from build123d import *

# Parameters (mm, degrees)
SKETCH1_W           = 47
SKETCH1_H           = 22
SKETCH1_R           = 5.25
BOSS_EXTRUDE1_DEPTH = 20
SKETCH2_R           = 10.5
SKETCH2_W           = 5.562030484
SKETCH2_H           = 6.723730134
CUT_EXTRUDE1_DEPTH  = 5


with BuildPart() as part:
    # Sketch1 → Boss-Extrude1 (new body)
    with BuildSketch(Plane.XY):
        Rectangle(SKETCH1_W, SKETCH1_H)
        Circle(SKETCH1_R, mode=Mode.SUBTRACT)
    extrude(amount=BOSS_EXTRUDE1_DEPTH)

    # Sketch2 → Cut-Extrude1 (cut)
    with BuildSketch(Plane.XZ.offset(11)):
        with BuildLine():
            ThreePointArc((3.201562119, 0), (7.43030884, 2.581070796), (10.004895252, 6.813768529))
            Line((10.004895252, 6.813768529), (10.004895252, 13.186231471))
            ThreePointArc((10.004895252, 13.186231471), (7.43030884, 17.418929204), (3.201562119, 20))
            Line((3.201562119, 20), (-3.201562119, 20))
            ThreePointArc((-3.201562119, 20), (-10.5, 10), (-3.201562119, 0))
            Line((-3.201562119, 0), (3.201562119, 0))
        make_face()
        with Locations((0, 10)):
            Circle(SKETCH2_R)
        with Locations((12.785910494, 10.175633596)):
            Rectangle(SKETCH2_W, SKETCH2_H)
        with BuildLine():
            Line((10.004895252, 13.186231471), (10.004895252, 6.813768529))
            ThreePointArc((10.004895252, 6.813768529), (10.375485534, 8.387765549), (10.5, 10))
            ThreePointArc((10.5, 10), (10.375485534, 11.612234451), (10.004895252, 13.186231471))
        make_face()
    extrude(amount=-CUT_EXTRUDE1_DEPTH, mode=Mode.SUBTRACT)


solid = part.part
Check sheet for the modelled part. Datum: model origin and axes. Units: mm. A direction names the side the tool comes from. Give positions to 0.01 mm unless a question says otherwise; leave off trailing zeros. Write each loop counter-clockwise with the first axis right and the second up, starting at its lowest first coordinate (ties: lowest second). Pieces come first, ordered by that corner, then holes. Notation, with made-up numbers: (9, -35.5) -> (28, -35.5) arc R6 ccw to (28, -30.5) -> close; hole circle Ø1 at (-9, 18.25). An arc over 180 degrees is marked (long way). One line per item, written item: value. Start each with the question number.
Item 1: Section check D-D on x = 13. Record the cut outline in (y, z), then the cut area to 3 significant figures.
Item 2: Draft check along Z on faces 3 (the flat face through (-6, 0, 0)), 4 (the flat face through (15.567, -9, 10)), 5 (the cylindrical face through (5, 1.6, 9.9)). Enter one of: +Z half, -Z half, draft (parallel to the pull), parting line (faces both ways), or undercut.
Item 3: Section check A-A on x = 0. Record the cut outline in (y, z), then the cut area to 3 significant figures.
Item 4: Section check C-C on z = 3.5. Record the cut outline in (x, y).
Item 5: Gauge pin test, flat ends, axial feed: pin 1 (6 mm diameter, centred on x = 4.5, z = 6, fed in from -Y); pin 2 (8.5 mm diameter, centred on x = 0, y = 0, fed in from -Z). Record the tip position at first contact, or that the pin passes through.
Item 6: Tool access check on faces 1 (the flat face through (0, 11, 10)), 2 (the flat face through (13, -9, 13.537)). Record the directions out of +Z, -Z, +X, -X, +Y, -Y that give a thin tool (end or side, any length) a straight path to the whole face; none if there is none.
Item 7: Material ranges on probe 1 along Y at (x, z) = (0, 6.5); probe 2 along Z at (x, y) = (7, -8); probe 3 along X at (y, z) = (-3.25, 7.25), recorded low to high. Write a range as from..to.
Item 8: Section check B-B on y = 0. Record the cut outline in (x, z).
Results list:
1. outline: (-11, 0) -> (11, 0) -> (11, 20) -> (-11, 20) -> (-11, 13.54) -> (-6, 13.54) -> (-6, 6.81) -> (-11, 6.81) -> close
1. area: 406 mm²
2. face 3: -Z half
2. face 4: undercut
2. face 5: draft
3. outline: (-6, 0) -> (-5.25, 0) -> (-5.25, 20) -> (-6, 20) -> close; (5.25, 0) -> (11, 0) -> (11, 20) -> (5.25, 20) -> close
3. area: 130 mm²
4. outline: (-23.5, -11) -> (-8.25, -11) -> (-8.25, -6) -> (8.25, -6) -> (8.25, -11) -> (23.5, -11) -> (23.5, 11) -> (-23.5, 11) -> close; hole circle Ø10.5 at (0, 0)
5. pin 1: y = -6
5. pin 2: through
6. face 1: +Z, -Z, +X, -X, +Y
6. face 2: -Y
7. probe 1: -6..-5.25, 5.25..11
7. probe 2: 0..2.17, 17.83..20
7. probe 3: -23.5..-4.12, 4.12..23.5
8. outline: (-23.5, 0) -> (-5.25, 0) -> (-5.25, 20) -> (-23.5, 20) -> close; (5.25, 0) -> (23.5, 0) -> (23.5, 20) -> (5.25, 20) -> close
